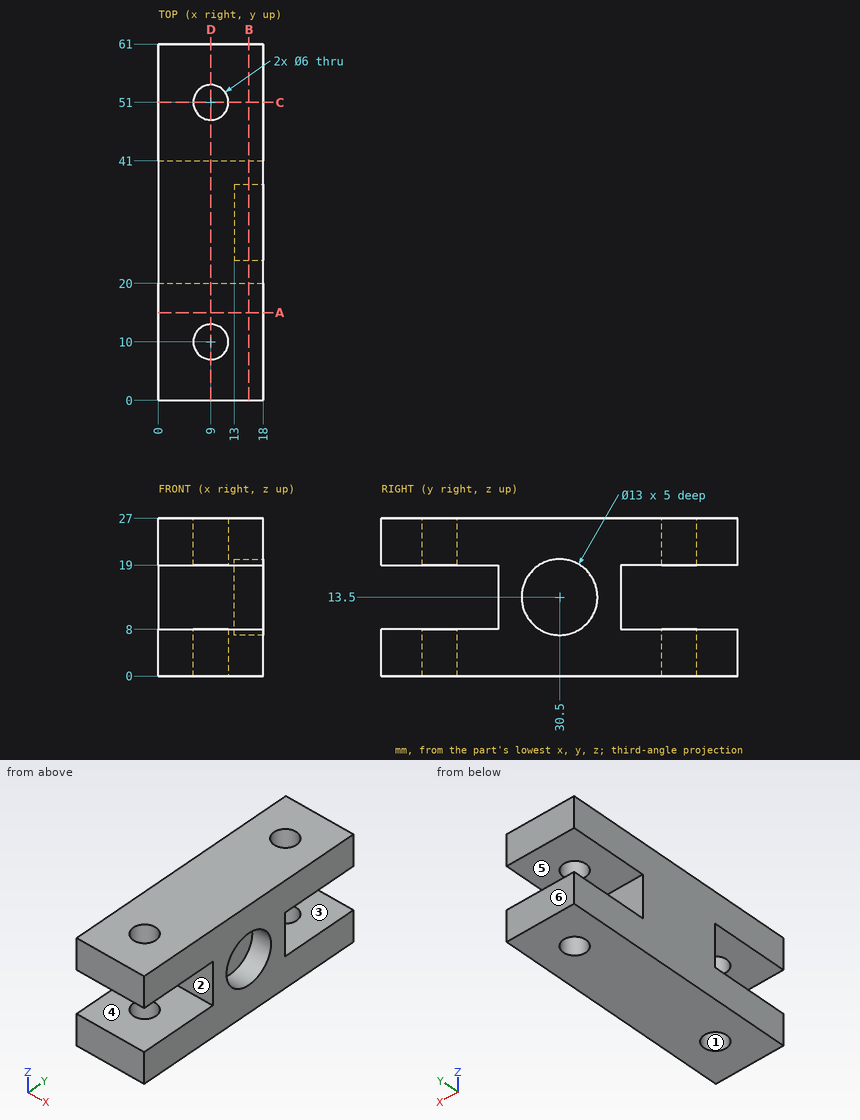
Answer from the drawing. Dimensions are ordinates in mm from the lowest x, y and z of the part. A direction names the side the tool comes from. Round coordinates to 2 decimals unless told otherwise and drop trailing zeros. Loops run counter-clockwise (first coordinate to the right, second up) from the corner with the lowest first, then second, coordinate; pieces in that order, holes last. Notation, with made-up numbers: (36.5, -36) - (82.5, -36) arc R20 cw to (82.5, -12) - close; hole circle Ø4 at (-18.75, -14.5). An arc over 180 degrees is marked (long way). Return JSON: item names as keys, results as strings. Group by question number.
1. The mould has two halves that part along Y. Classify the marked faces 1, 2 and 3: pulls with the +Y half, pulls with the -Y half, needs draft (parallel to the pull), parting line crosses it, or undercut.
2. The part is cut by section A-A on y = 15. Determine the outline of the cut face in (x, z).
3. The part is cut by section B-B on x = 15.5. Determine the outline of the cut face in (y, z), then the cut area to 3 significant figures.
4. The part is cut by section D-D on x = 9. Determine the outline of the cut face in (y, z), then the cut area to 4 significant figures.
5. Consider probe 1 along Y at (x, z) = (9, 3.25); probe 2 along Y at (x, z) = (16.45, 13.5); probe 3 along Z at (x, y) = (12, 4.5). Determine where each line is inside the solid, lowest interval first.
6. The part is cut by section C-C on y = 51. Determine the outline of the cut face in (x, z), then the cut area to 3 significant figures.
7. Which of the six approach directions +Z, -Z, +X, -X, +Y, -Y give full straight-line access (tool end or side, diameter ignored) to the marked faces 4, 5 and 6?
8. Each of these flat-tipped pins is pushed along its axis until it touches: P1, Ø5.5, axis at x = 12.5, z = 14, coming from the +Y side; P2, Ø7, axis at x = 9, y = 51, coming from the +Z side; P3, Ø11.5, axis at y = 30.5, z = 13.5, coming from the +X side; P4, Ø1, axis at x = 15.5, z = 12.5, coming from the -Y side. Where does it stop, or does it pass through?
Resolved:
{
 "1": {"face 1": "undercut", "face 2": "pulls with the -Y half", "face 3": "needs draft"},
 "2": {"outline": "(0, 0) - (18, 0) - (18, 8) - (0, 8) - close; (0, 19) - (18, 19) - (18, 27) - (0, 27) - close"},
 "3": {"outline": "(0, 0) - (61, 0) - (61, 8) - (41, 8) - (41, 19) - (61, 19) - (61, 27) - (0, 27) - (0, 19) - (20, 19) - (20, 8) - (0, 8) - close; hole circle Ø13 at (30.5, 13.5)", "area": "1,070 mm²"},
 "4": {"outline": "(0, 0) - (7, 0) - (7, 8) - (0, 8) - close; (0, 19) - (7, 19) - (7, 27) - (0, 27) - close; (13, 0) - (48, 0) - (48, 8) - (41, 8) - (41, 19) - (48, 19) - (48, 27) - (13, 27) - (13, 19) - (20, 19) - (20, 8) - (13, 8) - close; (54, 0) - (61, 0) - (61, 8) - (54, 8) - close; (54, 19) - (61, 19) - (61, 27) - (54, 27) - close", "area": "1,015 mm²"},
 "5": {"probe 1": "y = 0 to 7, 13 to 48, 54 to 61", "probe 2": "y = 20 to 24, 37 to 41", "probe 3": "z = 0 to 8, 19 to 27"},
 "6": {"outline": "(0, 0) - (6, 0) - (6, 8) - (0, 8) - close; (0, 19) - (6, 19) - (6, 27) - (0, 27) - close; (12, 0) - (18, 0) - (18, 8) - (12, 8) - close; (12, 19) - (18, 19) - (18, 27) - (12, 27) - close", "area": "192 mm²"},
 "7": {"face 4": "+X, -X, -Y", "face 5": "+X, -X, +Y", "face 6": "+Z, -Z, +X, -X, +Y"},
 "8": {"P1": "stops at y = 41", "P2": "stops at z = 27", "P3": "stops at x = 13", "P4": "stops at y = 20"}
}
